Can you work these out from the drawing? Everything is in mm from the part's minimum corner. A direction names the side the tool comes from. Coordinates: 2 decimals unless noted, no trailing zeros. Order: outer loops, then holes, each group sorted by start corner. A loop starts at its lowest first (then second) coordinate and runs counter-clockwise, first axis right, second up. Notation, with made-up numbers: (39.5, -17.5) -> (43.5, -17.5) arc R14 ccw to (43.5, -13.5) -> close; hole circle Ø7 at (56.5, 70). An arc over 180 degrees is marked (long way). Return JSON: item names as keys, results as strings. Group by question number.
1) If we section it at C-C, the plane x = 41: Please give me the cut outline in (y, z).
2) If we section it at D-D, the plane y = 23: Please give me the cut outline in (x, z).
3) For pin 1 (1 mm diameter, centred on x = 53, z = 4.5, fed in from +Y); pin 2 (0.6 mm diameter, centred on y = 53.5, z = 0.5, fed in from -X); pin 3 (12 mm diameter, centred on x = 11, y = 74.5, fed in from +Z), each with a flat end and sliding along its axis, tell me the tip position at first contact or that it passes through.
4) If I drill on probe 1 along Y at (x, z) = (52.85, 13); probe 2 along X at (y, z) = (13, 6); probe 3 along Z at (x, y) = (11.5, 81), over which ranges is the centre line in solid material (lowest first)? Write a range as from..to.
5) Thinking about a two-plate mould opening in X: for the marked faces 1, 2 and 3, which applies, +X half, -X half, draft (parallel to the pull), parting line (faces both ways), or undercut?
6) If we section it at A-A, the plane y = 5: Please give me the cut outline in (x, z), then the cut area to 3 significant figures.
7) For the marked faces 4 and 5, which set-ups out of +Z, -Z, +X, -X, +Y, -Y let a thin tool reach every point of the face, with its end or its side?
8) If we section it at B-B, the plane z = 8: Please give me the cut outline in (x, y), then the cut area to 3 significant figures.
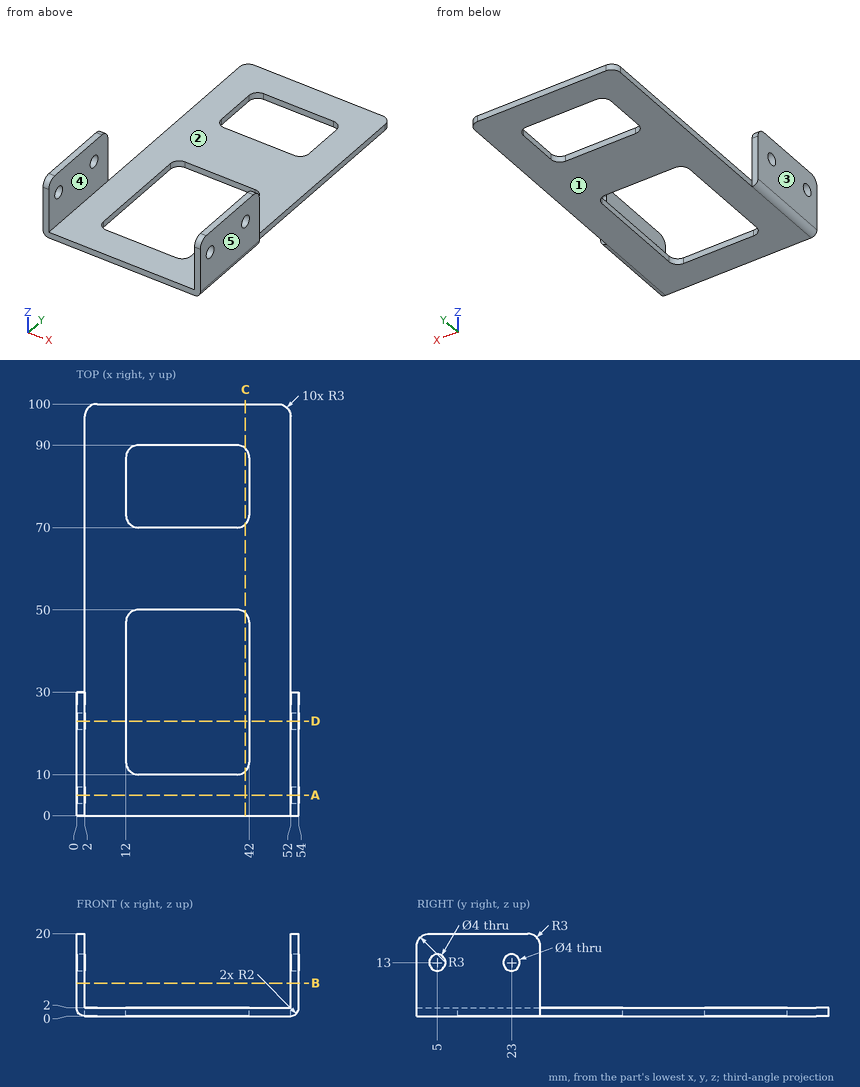
Result sheet:
{
 "1": {"outline": "(0, 0) -> (10.76, 0) -> (10.76, 2) -> (0, 2) -> close; (49.24, 0) -> (70.76, 0) -> (70.76, 2) -> (49.24, 2) -> close; (89.24, 0) -> (100, 0) -> (100, 2) -> (89.24, 2) -> close"},
 "2": {"outline": "(0, 2) arc R2 ccw to (2, 0) -> (12, 0) -> (12, 2) -> (2, 2) -> (2, 11) -> (0, 11) -> close; (0, 15) -> (2, 15) -> (2, 20) -> (0, 20) -> close; (42, 0) -> (52, 0) arc R2 ccw to (54, 2) -> (54, 11) -> (52, 11) -> (52, 2) -> (42, 2) -> close; (52, 15) -> (54, 15) -> (54, 20) -> (52, 20) -> close"},
 "3": {"pin 1": "stops at y = 30", "pin 2": "stops at x = 2", "pin 3": "stops at z = 2"},
 "4": {"probe 1": "y = 0..3, 7..21, 25..30", "probe 2": "x = 0..2, 52..54", "probe 3": "z = 0..2"},
 "5": {"face 1": "draft", "face 2": "undercut", "face 3": "-X half"},
 "6": {"outline": "(0, 2) arc R2 ccw to (2, 0) -> (52, 0) arc R2 ccw to (54, 2) -> (54, 11) -> (52, 11) -> (52, 2) -> (2, 2) -> (2, 11) -> (0, 11) -> close; (0, 15) -> (2, 15) -> (2, 20) -> (0, 20) -> close; (52, 15) -> (54, 15) -> (54, 20) -> (52, 20) -> close", "area": "162 mm2"},
 "7": {"face 4": "+Z, +Y, -Y", "face 5": "+Z, -Z, +X, +Y, -Y"},
 "8": {"outline": "(0, 0) -> (2, 0) -> (2, 30) -> (0, 30) -> close; (52, 0) -> (54, 0) -> (54, 30) -> (52, 30) -> close", "area": "120 mm2"}
}
